Part print with two shaded views. Sizes in mm from the minimum x, y, z corner. A direction names the side the tool comes from. Coordinates: 2 decimals unless noted, no trailing zeros. Order: outer loops, then holes, each group sorted by start corner. A loop starts at its lowest first (then second) coordinate and runs counter-clockwise, first axis right, second up. Notation, with made-up numbers: (28, -8.75) - (62, -8.75) arc R9 ccw to (62, 5.25) - close; hole circle Ø5 at (81, 39.25). An arc over 180 degrees is marked (long way). Return JSON: item names as keys, results as strings.
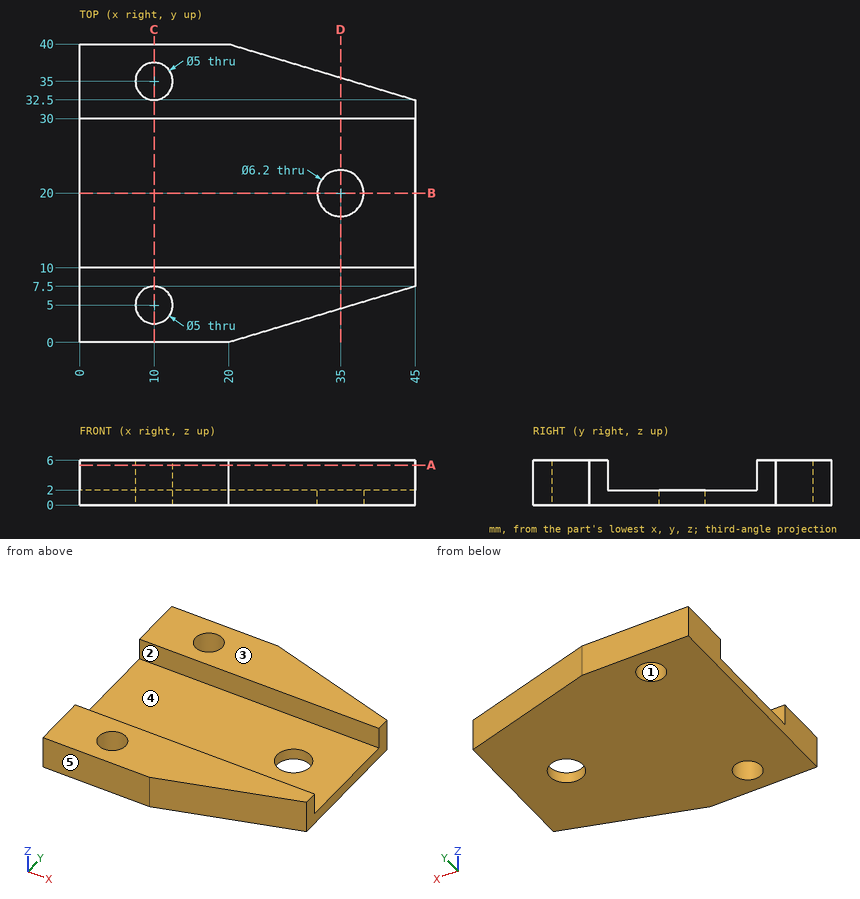
Item 1: Band-saw the part on C-C, the plane x = 10. List the corners of the cut face in (y, z).
Findings below:
{"outline": "(0, 0) - (2.5, 0) - (2.5, 6) - (0, 6) - close; (7.5, 0) - (32.5, 0) - (32.5, 6) - (30, 6) - (30, 2) - (10, 2) - (10, 6) - (7.5, 6) - close; (37.5, 0) - (40, 0) - (40, 6) - (37.5, 6) - close"}
Item 2: Mould opens along Y. For the marked faces 3, 4 and 5 say: released by +Y, released by -Y, zero draft, split by the parting line, or undercut.
Findings below:
{"face 3": "zero draft", "face 4": "undercut", "face 5": "released by -Y"}
Item 3: Band-saw the part on B-B, the plane y = 20. List the corners of the cut face in (x, z).
Findings below:
{"outline": "(0, 0) - (31.9, 0) - (31.9, 2) - (0, 2) - close; (38.1, 0) - (45, 0) - (45, 2) - (38.1, 2) - close"}
Item 4: Band-saw the part on D-D, the plane x = 35. List the corners of the cut face in (y, z).
Findings below:
{"outline": "(4.5, 0) - (16.9, 0) - (16.9, 2) - (10, 2) - (10, 6) - (4.5, 6) - close; (23.1, 0) - (35.5, 0) - (35.5, 6) - (30, 6) - (30, 2) - (23.1, 2) - close"}
Item 5: Drop flat-ended pins along their axis: P1, Ø1.2, axis at x = 33.5, z = 3, coming from the +Y side; P2, Ø3, axis at x = 28.5, z = 3.5, coming from the -Y side; P3, Ø3, axis at x = 22.5, z = 1.5, coming from the -Y side. Give the stop position or say it passes through.
Findings below:
{"P1": "stops at y = 36.13", "P2": "stops at y = 2.1", "P3": "stops at y = 0.3"}
Item 6: Band-saw the part on A-A, the plane z = 5.35. List the corners of the cut face in (x, y).
Findings below:
{"outline": "(0, 0) - (20, 0) - (45, 7.5) - (45, 10) - (0, 10) - close; (0, 30) - (45, 30) - (45, 32.5) - (20, 40) - (0, 40) - close; hole circle Ø5 at (10, 5); hole circle Ø5 at (10, 35)"}
Item 7: Which spindle directions (+Z, -Z, +X, -X, +Y, -Y) get a long thin tool onto all of the face, cutting with end or side? Do the marked faces 1 and 2. Say none if no direction does.
Findings below:
{"face 1": "+Z, -Z", "face 2": "+Z, +X, -X"}
Item 8: Wall check: L1, parallel to Y at x = 10, z = 2.85; L2, parallel to Y at x = 10, z = 1.2; L3, parallel to Y at x = 13, z = 2.95. Give the ranges that are in metal, low to high. Write a range as [from, to].
Findings below:
{"L1": "y = [0, 2.5], [7.5, 10], [30, 32.5], [37.5, 40]", "L2": "y = [0, 2.5], [7.5, 32.5], [37.5, 40]", "L3": "y = [0, 10], [30, 40]"}
